```python
from build123d import *

# Parameters (mm, degrees)
F2_R     = 8.73125
F3_DEPTH = 6.35


with BuildPart() as f1:
    # F0 (on Right) → F1 (revolve)
    with BuildSketch(Plane.YZ):
        Polygon((-14.680734, 9.332753), (-27.380734, 2.729445), (-27.380734, 0.187998), (-26.010094, 0.187998), (-26.010094, -1.148191), (-27.371027, -1.148191), (-27.380734, -3.620555), (-14.680734, -3.620555), align=None)
    revolve(axis=Axis((0, -14.680734, 2.856099), (0, 0, -1)))

    # F2 (on face) → F3 (cut)
    with BuildSketch(Plane(origin=(0, 0, -3.620555), x_dir=(1, 0, 0), z_dir=(0, 0, -1))):
        with Locations((0, 14.680734)):
            Circle(F2_R)
    extrude(amount=-F3_DEPTH, mode=Mode.SUBTRACT)


solid = f1.part
```
Check sheet for the modelled part. Datum: model origin and axes. Units: mm. A direction names the side the tool comes from. Round coordinates to 2 decimals unless told otherwise and drop trailing zeros. Order: outer loops, then holes, each group sorted by start corner. A loop starts at its lowest first (then second) coordinate and runs counter-clockwise, first axis right, second up. Notation, with made-up numbers: M 23,80 L 80,80 A13 ccw 80,100 Z; hole C 10,6 d5. An arc over 180 degrees is marked long. Answer in a Markdown table with one row per item.
(1) Gauge pin test, flat ends, axial feed: pin 1 (3 mm diameter, centred on x = 5.5, y = -8.5, fed in from +Z); pin 2 (6 mm diameter, centred on y = -18, z = 1.5, fed in from +X); pin 3 (4 mm diameter, centred on x = 0, y = -10.5, fed in from +Z); pin 4 (1 mm diameter, centred on y = -23.5, z = 6.5, fed in from -X). Record the tip position at first contact, or that the pin passes through.
Findings:
| item | result |
|---|---|
| pin 1 | stops at z = 5.81 |
| pin 2 | stops at x = 12.7 |
| pin 3 | stops at z = 8.2 |
| pin 4 | passes through |
(2) Section check B-B on z = 6.5. Record the boundary of the cut face in (x, y).
Findings:
| item | result |
|---|---|
| outline | C 0,-14.68 d10.9 |
(3) Material ranges on line 1 along Y through (x, z) = (0, 0.75); line 2 along Y through (x, z) = (0, -1); line 3 along Z through (x, y) = (-11.25, -16.25), recorded low to high. Write a range as from..to.
Findings:
| item | result |
|---|---|
| line 1 | y = -27.38..-23.41, -5.95..-1.98 |
| line 2 | y = -26.01..-23.41, -5.95..-3.35 |
| line 3 | z = -3.62..-1.15, 0.19..3.43 |
(4) Set-up check for faces 1 (the conical face through (-0.03, -13.89, 8.92)), 2 (the flat face through (-8, -23, -1.148)), 3 (the flat face through (0, -15, 2.729)): record each of +Z, -Z, +X, -X, +Y, -Y from which the full face is reachable in a straight line by a thin tool's end or side.
Findings:
| item | result |
|---|---|
| face 1 | +Z |
| face 2 | none |
| face 3 | -Z |
(5) Draft check along Z on faces 4 (the cylindrical face through (-1.893, -6.157, -0.49)), 5 (the cylindrical face through (-3.403, -25.487, -0.489)), 6 (the flat face through (0, -3, 0.188)). Enter one of: +Z half, -Z half, draft (parallel to the pull), parting line (faces both ways), or undercut.
Findings:
| item | result |
|---|---|
| face 4 | draft |
| face 5 | undercut |
| face 6 | undercut |
(6) Section check A-A on z = -1.75. Record the boundary of the cut face in (x, y).
Findings:
| item | result |
|---|---|
| outline | C 0,-14.68 d25.39; hole C 0,-14.68 d17.46 |
(7) Section check C-C on z = 2.25. Record the boundary of the cut face in (x, y).
Findings:
| item | result |
|---|---|
| outline | C 0,-14.68 d25.4; hole C 0,-14.68 d17.46 |
